```python
from build123d import *

# Parameters (mm, degrees)
SKETCH_1_R      = 1
EXTRUDE_1_DEPTH = 2
SKETCH_2_R      = 2
EXTRUDE_2_DEPTH = 7


with BuildPart() as part:
    # 草图1 → 凸台-拉伸1 (new body)
    with BuildSketch(Plane(origin=(0, 0, 0), x_dir=(1, 0, 0), z_dir=(0, 1, 0))):
        with Locations(Location((0, 0, 0), (0, 0, 270))):
            Circle(SKETCH_1_R)
    extrude(amount=EXTRUDE_1_DEPTH)

    # 草图2 → 凸台-拉伸2 (add)
    with BuildSketch(Plane(origin=(0, 2, 0), x_dir=(1, 0, 0), z_dir=(0, 1, 0))):
        with Locations(Location((0, 0, 0), (0, 0, 270))):
            Circle(SKETCH_2_R)
    extrude(amount=EXTRUDE_2_DEPTH)

    # 草图3 → 旋转1 (revolve)
    with BuildSketch(Plane.XY, mode=Mode.PRIVATE) as revolve_1_sk:
        Polygon((0, 9), (0, 7), (2.2, 7.5), (2.2, 8.5), align=None)
    revolve(revolve_1_sk.sketch.rotate(Axis((0, 9, 0), (0, -1, 0)), 90), axis=Axis((0, 9, 0), (0, -1, 0)))


solid = part.part
```
Input: part model. Units: mm. Frame: model coordinates. A direction names the side the tool comes from. Coordinates: 2 decimals unless noted, no trailing zeros. Write each loop counter-clockwise with the first axis right and the second up, starting at its lowest first coordinate (ties: lowest second). Pieces come first, ordered by that corner, then holes.
1) Section B-B on x = 0. Output: boundary loops of the cut face in (y, z), and give its area (3 significant figures).
2) Section A-A on z = 0. Output: boundary loops of the cut face in (x, y).
3) Pin query (flat end, axial travel): pin 1 Ø1 at (y, z) = (5.5, 1) entering from -X. Return the tip coordinate at first contact, or that it passes through.
4) Section D-D on y = 0.5. Output: boundary loops of the cut face in (x, z).
5) Section C-C on y = 3.75. Output: boundary loops of the cut face in (x, z).
6) Set-up query: faces 1 (the cylindrical face through (-2, 5, 0)), 2 (the cylindrical face through (-1.952, 8.77, -0.434)), 3 (the flat face through (0, 0, 0)). Return all of +Z, -Z, +X, -X, +Y, -Y with unobstructed straight access to the full face (end or side cutting, diameter ignored); none if empty.
7) Material intervals for line 1 along Y through (x, z) = (1.5, 0.75); line 2 along X through (y, z) = (2.75, 0.75); line 3 along Y through (x, z) = (1.1, -1.8), sorted ascending.
Check result:
1. outline: (0, -1) - (2, -1) - (2, -2) - (7.45, -2) - (7.5, -2.2) - (8.5, -2.2) - (8.55, -2) - (9, -2) - (9, 2) - (8.55, 2) - (8.5, 2.2) - (7.5, 2.2) - (7.45, 2) - (2, 2) - (2, 1) - (0, 1) - close
1. area: 32.4 mm2
2. outline: (-2.2, 7.5) - (-2, 7.45) - (-2, 2) - (-1, 2) - (-1, 0) - (1, 0) - (1, 2) - (2, 2) - (2, 7.45) - (2.2, 7.5) - (2.2, 8.5) - (2, 8.55) - (2, 9) - (-2, 9) - (-2, 8.55) - (-2.2, 8.5) - close
3. pin 1: stops at x = -1.94
4. outline: circle Ø2 at (0, 0)
5. outline: circle Ø4 at (0, 0)
6. face 1: -Y
6. face 2: +Y
6. face 3: +Z, -Z, +X, -X, -Y
7. line 1: y = 2 to 9
7. line 2: x = -1.85 to 1.85
7. line 3: y = 7.48 to 8.52
